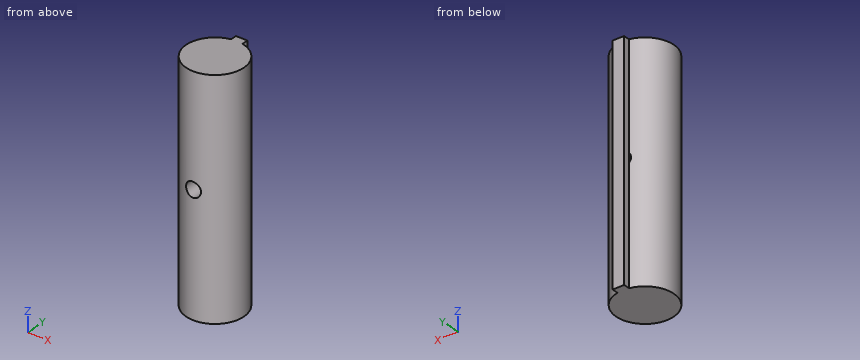
```python
from build123d import *

# Parameters (mm, degrees)
SKETCH1_R               = 6.35
BOSS_EXTRUDE1_DEPTH     = 50.8
CUT_EXTRUDE1_DEPTH      = 52.587643869
CUT_EXTRUDE1_DEPTH_BACK = 52.587643869
SKETCH2_R               = 1.643209115
BOSS_EXTRUDE2_START     = -50.8
BOSS_EXTRUDE2_DEPTH     = 50.8


with BuildPart() as part:
    # Sketch1 → Boss-Extrude1 (new body)
    with BuildSketch(Plane.XY):
        Circle(SKETCH1_R)
    extrude(amount=BOSS_EXTRUDE1_DEPTH)

    # Sketch2 → Cut-Extrude1 (cut, two sides: drawn at the far end of the back side and taken through both)
    with BuildSketch(Plane(origin=(0, 0, 0), x_dir=(1, 0, 0), z_dir=(0, 1, 0)).offset(-CUT_EXTRUDE1_DEPTH_BACK)):
        with Locations(Location((0, -26.623855977, 0), (0, 0, 270))):
            Circle(SKETCH2_R)
    extrude(amount=CUT_EXTRUDE1_DEPTH + CUT_EXTRUDE1_DEPTH_BACK, mode=Mode.SUBTRACT)

    # Sketch4 → Boss-Extrude2 (add)
    with BuildSketch(Plane.XY.offset(50.8).offset(BOSS_EXTRUDE2_START)):
        with BuildLine():
            Line((-1.27, 6.221703947), (-1.27, 7.62))
            Line((-1.27, 7.62), (1.27, 7.62))
            Line((1.27, 7.62), (1.27, 6.221703947))
            ThreePointArc((1.27, 6.221703947), (0, 6.35), (-1.27, 6.221703947))
        make_face()
    extrude(amount=BOSS_EXTRUDE2_DEPTH)


solid = part.part
```
The listing builds one solid part. Answer for the finished solid, in the listing's coordinates (mm). Give positions to 0.01 mm unless a question says otherwise; leave off trailing zeros. Order: outer loops, then holes, each group sorted by start corner. A loop starts at its lowest first (then second) coordinate and runs counter-clockwise, first axis right, second up. Notation, with made-up numbers: (-31, 52) -> (12, 52) arc R19 ccw to (12, 66) -> close; hole circle Ø2 at (1, 45). An arc over 180 degrees is marked (long way). Answer as a JSON object with one key per item and string values. Group by question number.
Item 1: The part is cut by section A-A on x = 0. Write down the section's boundary in (y, z), and give its area (3 significant figures).
Item 2: Consider L1, parallel to Z at x = 0, y = 1.5; L2, parallel to X at y = 6.5, z = 6.5; L3, parallel to Z at x = 1, y = -4.25. Determine where each line is inside the solid, lowest interval first. Write a range as from..to.
Item 3: The part is cut by section C-C on z = 45. Write down the section's boundary in (x, y).
Item 4: Flat-ended cylindrical pins translate along their axes: pin 1 (1.5 mm diameter, centred on x = -3, z = 15.5, fed in from -Y); pin 2 (4 mm diameter, centred on y = -3, z = 23, fed in from -X); pin 3 (2 mm diameter, centred on x = 3.5, z = 5.5, fed in from -Y). Find the tip coordinate at first contact, or state that the pin passes through.
Item 5: The part is cut by section B-B on y = -1.75. Write down the section's boundary in (x, z).
Item 6: The part is cut by section D-D on y = -4. Write down the section's boundary in (x, z).
Result set:
{
 "1": {"outline": "(-6.35, 0) -> (7.62, 0) -> (7.62, 50.8) -> (-6.35, 50.8) -> (-6.35, 28.27) -> (6.35, 28.27) -> (6.35, 24.98) -> (-6.35, 24.98) -> close", "area": "668 mm²"},
 "2": {"L1": "0..24.98, 28.27..50.8", "L2": "-1.27..1.27", "L3": "0..25.32, 27.93..50.8"},
 "3": {"outline": "(-1.27, 6.22) arc R6.35 ccw (long way) to (1.27, 6.22) -> (1.27, 7.62) -> (-1.27, 7.62) -> close"},
 "4": {"pin 1": "y = -5.94", "pin 2": "x = -6.27", "pin 3": "y = -5.84"},
 "5": {"outline": "(-6.1, 0) -> (6.1, 0) -> (6.1, 50.8) -> (-6.1, 50.8) -> close; hole circle Ø3.29 at (0, 26.62)"},
 "6": {"outline": "(-4.93, 0) -> (4.93, 0) -> (4.93, 50.8) -> (-4.93, 50.8) -> close; hole circle Ø3.29 at (0, 26.62)"}
}
